Geometry: final body of the model. Coordinates: model frame, mm. Coordinates: 2 decimals unless noted, no trailing zeros. Loops run counter-clockwise (first coordinate to the right, second up) from the corner with the lowest first, then second, coordinate; pieces in that order, holes last. Notation, with made-up numbers: (61.5, -38) - (111.5, -38) arc R15 cw to (111.5, -29) - close; hole circle Ø10 at (-10, 82.25). An arc over 180 degrees is marked (long way). Answer in a Markdown table with one row per item.
from build123d import *

# Parameters (mm, degrees)
F0_W     = 71.12
F0_H     = 137.16
F1_DEPTH = 22.86
F2_W     = 12.7
F2_H     = 5.08
F3_DEPTH = 11.43
F4_W     = 7.62
F4_H     = 5.08
F5_DEPTH = 3.81


with BuildPart() as f1:
    # F0 (on Top) → F1 (new body)
    with BuildSketch(Plane.XY):
        with Locations((-15.782022, -0.143904)):
            Rectangle(F0_W, F0_H)
    extrude(amount=F1_DEPTH)

    # F2 (on face) → F3 (cut)
    with BuildSketch(Plane(origin=(0, 68.436096, 0), x_dir=(-1, 0, 0), z_dir=(0, 1, 0))):
        with Locations((-5.807978, 10.16)):
            Rectangle(F2_W, F2_H)
        with Locations((37.372022, 10.16)):
            Rectangle(F2_W, F2_H)
    extrude(amount=-F3_DEPTH, mode=Mode.SUBTRACT)

    # F4 (on face) → F5 (cut)
    with BuildSketch(Plane.YZ.offset(19.777978)):
        with Locations((35.416096, 11.43)):
            Rectangle(F4_W, F4_H)
    extrude(amount=-F5_DEPTH, mode=Mode.SUBTRACT)


solid = f1.part
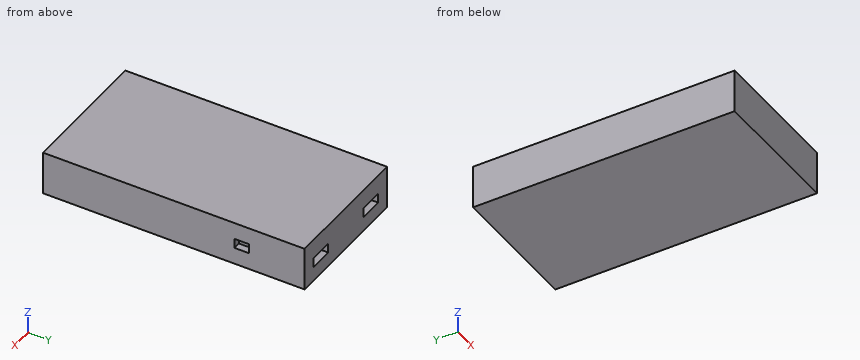
(1) Cut plane B-B on x = 5.5. Output: boundary loops of the cut face in (y, z).
Verdict:
| item | result |
|---|---|
| outline | (-68.72, 0) - (68.44, 0) - (68.44, 7.62) - (57.01, 7.62) - (57.01, 12.7) - (68.44, 12.7) - (68.44, 22.86) - (-68.72, 22.86) - close |
(2) First-contact query: pin 1 Ø2.5 at (x, z) = (7, 9) entering from +Y. Flat tip, straight axial feed; report the tip coordinate or a pass-through.
Verdict:
| item | result |
|---|---|
| pin 1 | stops at y = 57.01 |
(3) Ray query, probe 1 along Z at (x, y) = (-32.5, 60); probe 2 along Y at (x, z) = (10, 10.75). Return the intervals inside material, ascending.
Verdict:
| item | result |
|---|---|
| probe 1 | z = 0 to 7.62, 12.7 to 22.86 |
| probe 2 | y = -68.72 to 57.01 |
(4) Cut plane A-A on y = 59.5. Output: boundary loops of the cut face in (x, z), then the cut area to 3 significant figures.
Verdict:
| item | result |
|---|---|
| outline | (-51.34, 0) - (19.78, 0) - (19.78, 22.86) - (-51.34, 22.86) - close; hole (-43.72, 7.62) - (-31.02, 7.62) - (-31.02, 12.7) - (-43.72, 12.7) - close; hole (-0.54, 7.62) - (12.16, 7.62) - (12.16, 12.7) - (-0.54, 12.7) - close |
| area | 1,500 mm² |
